Can you work these out from the model? Positions are in its coordinate system, mm. A direction names the side the tool comes from. Round coordinates to 2 decimals unless told otherwise and drop trailing zeros. Loops run counter-clockwise (first coordinate to the right, second up) from the corner with the lowest first, then second, coordinate; pieces in that order, holes last.
from build123d import *

# Parameters (mm, degrees)
Y_KSEKLIK_EKSTR_ZYON1_DEPTH      = 220
Y_KSEKLIK_EKSTR_ZYON1_DEPTH_BACK = 220
IZIM1_W                          = 26
IZIM1_H                          = 26


with BuildPart() as part:
    # Çizim1 → Yükseklik-Ekstrüzyon1 (new, two sides: drawn at the far end of the back side and taken through both)
    with BuildSketch(Plane.XY.offset(-Y_KSEKLIK_EKSTR_ZYON1_DEPTH_BACK)):
        with BuildLine():
            Line((-13, 15), (13, 15))
            ThreePointArc((13, 15), (14.414213562, 14.414213562), (15, 13))
            Line((15, 13), (15, -13))
            ThreePointArc((15, -13), (14.414213562, -14.414213562), (13, -15))
            Line((13, -15), (-13, -15))
            ThreePointArc((-13, -15), (-14.414213562, -14.414213562), (-15, -13))
            Line((-15, -13), (-15, 13))
            ThreePointArc((-15, 13), (-14.414213562, 14.414213562), (-13, 15))
        make_face()
        Rectangle(IZIM1_W, IZIM1_H, mode=Mode.SUBTRACT)
    extrude(amount=Y_KSEKLIK_EKSTR_ZYON1_DEPTH + Y_KSEKLIK_EKSTR_ZYON1_DEPTH_BACK)


solid = part.part
(1) If we mould it in two halves opening along X, with no side actions, what happens to faces 3 (the flat face through (0, 15, -3)), 4 (the flat face through (-15, 0, -3)), 5 (the flat face through (0, -13, -3))? For each: released by +X, released by -X, zero draft, split by the parting line, or undercut.
Worked answers:
face 3: zero draft
face 4: released by -X
face 5: undercut
(2) If we section it at A-A, the plane y = -4.75: List the corners of the cut face in (x, z) for me.
Worked answers:
outline: (-15, -220) - (-13, -220) - (-13, 220) - (-15, 220) - close; (13, -220) - (15, -220) - (15, 220) - (13, 220) - close
(3) If we section it at C-C, the plane z = -168: List the corners of the cut face in (x, y) for me, then the cut area to 3 significant figures.
Worked answers:
outline: (-15, -13) arc R2 ccw to (-13, -15) - (13, -15) arc R2 ccw to (15, -13) - (15, 13) arc R2 ccw to (13, 15) - (-13, 15) arc R2 ccw to (-15, 13) - close; hole (-13, -13) - (13, -13) - (13, 13) - (-13, 13) - close
area: 221 mm2
(4) Will this pin go through, and if not, where does the flat tip stop? P1, Ø6, axis at x = 4.5, y = -7.5, coming from the -Z side.
Worked answers:
P1: passes through
(5) For faces 1 (the flat face through (-13, 0, -3)), 2 (the flat face through (15, 0, -3)), which set-ups out of +Z, -Z, +X, -X, +Y, -Y let a thin tool reach every point of the face, with its end or its side?
Worked answers:
face 1: +Z, -Z
face 2: +Z, -Z, +X, +Y, -Y
(6) If I drill on line 1 (Y direction, x = -0.25, z = 0); line 2 (Y direction, x = -13.25, z = 147.5), over which ranges is the centre line in solid material (lowest first)?
Worked answers:
line 1: y = -15 to -13, 13 to 15
line 2: y = -14.98 to 14.98
